Job drawing, mm, ordinate dimensions from the low corner. One solid piece. Give positions to 0.01 mm unless a question says otherwise; leave off trailing zeros. Order: outer loops, then holes, each group sorted by start corner. A loop starts at its lowest first (then second) coordinate and runs counter-clockwise, first axis right, second up. Notation, with made-up numbers: (79.25, -19.75) -> (91.25, -19.75) arc R19 ccw to (91.25, -10.75) -> close; hole circle Ø10 at (-30, 75.25). An arc over 180 degrees is marked (long way). Write item = value, one per line. Start each with the question number.
(1) Flat gauge pin, fed straight in: pin 1 (3.5 mm diameter, centred on x = 61.12, y = 172.62, fed in from +Z) (1 decimal). Where does the tip first touch, or does it go through?
(2) Probe line 1 along Y through (x, z) = (44.45, 4.5); line 2 along X through (y, z) = (10, 3.5); line 3 along X through (y, z) = (173, 5.25) (1 decimal). List the from-to ranges inside material, lowest first. Write a range as from..to.
(3) Saw through at A-A, the plane x = 44.45. List the corners of the cut face in (y, z), then the cut area to 3 significant figures.
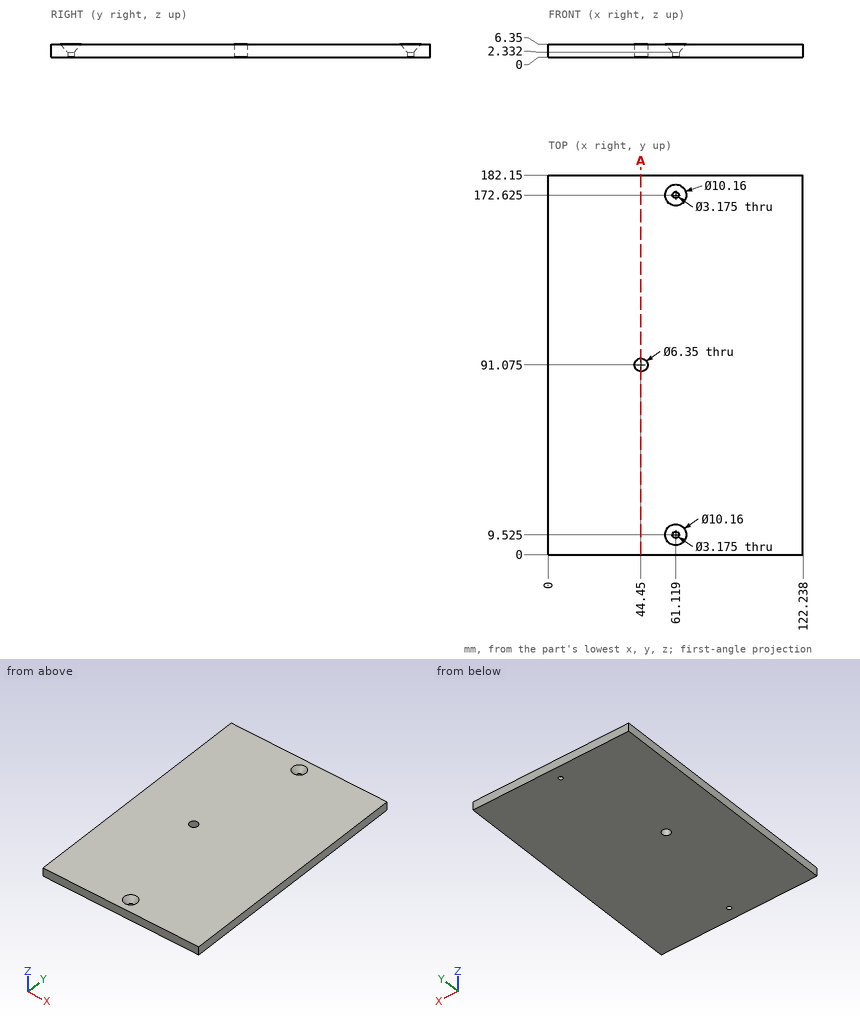
Results list:
q1.pin_1 = 2.5
q2.line_1 = 0..87.9, 94.25..182.15
q2.line_2 = 0..58.56, 63.68..122.24
q2.line_3 = 0..57, 65.2..122.2
q3.outline = (0, 0) -> (87.9, 0) -> (87.9, 6.35) -> (0, 6.35) -> close; (94.25, 0) -> (182.15, 0) -> (182.15, 6.35) -> (94.25, 6.35) -> close
q3.area = 1,120 mm^2
